Here's how the part is built. I have some questions about the finished solid (model axes, mm). Face numbers are marked on the shaded views. A direction names the side the tool comes from. Round coordinates to 2 decimals unless told otherwise and drop trailing zeros. Write each loop counter-clockwise with the first axis right and the second up, starting at its lowest first coordinate (ties: lowest second). Pieces come first, ordered by that corner, then holes. Notation, with made-up numbers: (-17, 30) - (4, 30) arc R33 ccw to (4, 62) - close; hole circle Ø6 at (38, 76). An arc over 180 degrees is marked (long way). Use one line per item in the form item = value. Start each with the question number.
1. I want a section at B-B, the plane y = -14.45. List the corners of the cut face in (x, z) for me, plus the area to 3 significant figures.
2. I want a section at D-D, the plane x = 12.5. List the corners of the cut face in (y, z) for me.
3. If I drill on line 1 along Y through (x, z) = (4, 3.05); line 2 along X through (y, z) = (-80, 105.25); line 3 along Y through (x, z) = (22, 2.75), over which ranges is the centre line in solid material (lowest first)?
4. I want a section at C-C, the plane z = 14.5. List the corners of the cut face in (x, y) for me.
5. Which directions (+Z, -Z, +X, -X, +Y, -Y) give clear straight access to the entire face, cutting with the end or side of a thin tool? Please do the marked faces 1 and 2.
6. I want a section at A-A, the plane x = 22. List the corners of the cut face in (y, z) for me, plus the area to 3 significant figures.
7. Will these pins go through, and if not, where does the flat tip stop? pin 1 (1.2 mm diameter, centred on x = 11.5, z = 3, fed in from -Y); pin 2 (2 mm diameter, centred on x = 4, y = -4.45, fed in from +Z) (3 decimals); pin 3 (10 mm diameter, centred on x = 35, z = 14.5, fed in from +Y); pin 4 (3 mm diameter, centred on x = 26.5, y = -51.5, fed in from -Z).
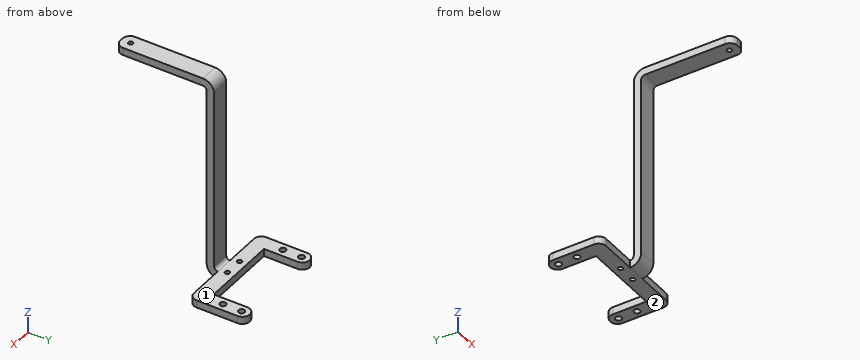
```python
from build123d import *

# Parameters (mm, degrees)
EXTRUDE_1_DEPTH                  = 3
SHEET_METAL_1_OUTLINE_W          = 8
SHEET_METAL_1_OUTLINE_H          = 1
SHEET_METAL_1_DEPTH              = 57.5
SHEET_METAL_1_2_OUTLINE_W        = 22
SHEET_METAL_1_2_OUTLINE_H        = 1
SHEET_METAL_1_2_DEPTH            = 8
SHEET_START                      = 49.5
SHEET_METAL_1_3_OUTLINE_W        = 22
SHEET_METAL_1_3_OUTLINE_H        = 1
SHEET_METAL_1_3_DEPTH            = 8
SM_EDGE_FLANGE_1_DEPTH           = 10
SM_EDGE_FLANGE_2_STRIP_W         = 20
SM_EDGE_FLANGE_2_STRIP_H         = 4
SM_EDGE_FLANGE_2_STRIP_CUT_DEPTH = 10
SM_EDGE_FLANGE_2_DEPTH           = 10
FILLET_1_R                       = 4
M4X0_7_1_D                       = 3.3
M3X0_5_1_D                       = 2.5
M3X0_5_2_D                       = 2.5


# Read off the part's stored shape, not the designer's step: 轉換-實體1
# Sheet-metal steps are written as plain solids
with BuildPart() as part:
    # Sketch 1 → 填料-伸長1 (new body)
    with BuildSketch(Plane.XY):
        Polygon((8, 0), (8, -22), (49.5, -22), (49.5, 0), (57.5, 0), (57.5, -30), (8, -30), (0, -30), (0, 0), align=None)
    extrude(amount=EXTRUDE_1_DEPTH)

    # Sheet Metal 1 outline → Sheet Metal 1 (add)
    with BuildSketch(Plane.YZ):
        with Locations((-26, 3.5)):
            Rectangle(SHEET_METAL_1_OUTLINE_W, SHEET_METAL_1_OUTLINE_H)
    extrude(amount=SHEET_METAL_1_DEPTH)

    # Sheet Metal 1 2 outline → Sheet Metal 1 2 (add)
    with BuildSketch(Plane.YZ):
        with Locations((-11, 3.5)):
            Rectangle(SHEET_METAL_1_2_OUTLINE_W, SHEET_METAL_1_2_OUTLINE_H)
    extrude(amount=SHEET_METAL_1_2_DEPTH)

    # Sheet Metal 1 3 outline → Sheet Metal 1 3 (add)
    with BuildSketch(Plane.YZ.offset(SHEET_START)):
        with Locations((-11, 3.5)):
            Rectangle(SHEET_METAL_1_3_OUTLINE_W, SHEET_METAL_1_3_OUTLINE_H)
    extrude(amount=SHEET_METAL_1_3_DEPTH)

    # 邊線-凸緣1 section (across the edge) → 邊線-凸緣1 (add)
    with BuildSketch(Plane(origin=(23.75, -32, 4), x_dir=(0, 1, 0), z_dir=(1, 0, 0))):
        with BuildLine():
            Line((-4, 2), (-4, 104.15))
            Line((-4, 104.15), (0, 104.15))
            Line((0, 104.15), (0, 2))
            ThreePointArc((0, 2), (0.585786438, 0.585786438), (2, 0))
            Line((2, 0), (2, -4))
            ThreePointArc((2, -4), (-2.242640687, -2.242640687), (-4, 2))
        make_face()
    extrude(amount=SM_EDGE_FLANGE_1_DEPTH)

    # 邊線-凸緣2 strip (across the edge) → 邊線-凸緣2 strip cut (cut)
    with BuildSketch(Plane(origin=(33.75, -36, 108.15), x_dir=(0, 0, -1), z_dir=(-1, 0, 0))):
        with Locations((-4, -2)):
            Rectangle(SM_EDGE_FLANGE_2_STRIP_W, SM_EDGE_FLANGE_2_STRIP_H)
    extrude(amount=SM_EDGE_FLANGE_2_STRIP_CUT_DEPTH, mode=Mode.SUBTRACT)

    # 邊線-凸緣2 section (across the edge) → 邊線-凸緣2 (add)
    with BuildSketch(Plane(origin=(33.75, -36, 108.15), x_dir=(0, 0, -1), z_dir=(-1, 0, 0))):
        with BuildLine():
            Line((0, 2), (0, 49))
            Line((0, 49), (4, 49))
            Line((4, 49), (4, 2))
            ThreePointArc((4, 2), (4.585786438, 0.585786438), (6, 0))
            Line((6, 0), (6, -4))
            ThreePointArc((6, -4), (1.757359313, -2.242640687), (0, 2))
        make_face()
    extrude(amount=SM_EDGE_FLANGE_2_DEPTH)

    # 圓角1
    fillet_1_edges = [part.edges().sort_by_distance(p)[0] for p in [
        (0, -30, 2),
        (57.5, -30, 2),
        (57.5, 0, 2),
        (49.5, 0, 2),
        (8, 0, 2),
        (0, 0, 2),
        (33.75, -85, 106.15),
        (23.75, -85, 106.15),
    ]]
    fillet(fillet_1_edges, radius=FILLET_1_R - 0.0001)  # a hair under: the kernel refuses the full size

    # M4x0.7 螺紋孔1 (through all)
    with Locations(Plane(origin=(53.5, -4.45, 0), x_dir=(-1, 0, 0), z_dir=(0, 0, -1))):
        with Locations((0, 0), (0, -10), (49.5, -10), (49.5, 0)):
            Hole(M4X0_7_1_D / 2)

    # M3x0.5 螺紋孔1 (through all)
    with Locations(Plane(origin=(28.75, -80, 104.15), x_dir=(-1, 0, 0), z_dir=(0, 0, -1))):
        with Locations((0, 0)):
            Hole(M3X0_5_1_D / 2)

    # M3x0.5 螺紋孔2 (through all)
    with Locations(Plane(origin=(22, -26, 0), x_dir=(-1, 0, 0), z_dir=(0, 0, -1))):
        with Locations((0, 0), (-10, 0)):
            Hole(M3X0_5_2_D / 2)


solid = part.part
```
Model answer:
q1.outline = (0, 0) - (2.35, 0) - (2.35, 4) - (0, 4) - close; (5.65, 0) - (8, 0) - (8, 4) - (5.65, 4) - close; (49.5, 0) - (51.85, 0) - (51.85, 4) - (49.5, 4) - close; (55.15, 0) - (57.5, 0) - (57.5, 4) - (55.15, 4) - close
q1.area = 37.6 mm2
q2.outline = (-30, 0) - (-22, 0) - (-22, 4) - (-30, 4) - close
q3.line_1 = -30 to -16.1, -12.8 to -6.1, -2.8 to 0
q3.line_2 = 23.75 to 27.5, 30 to 33.75
q3.line_3 = -30 to -27.25, -24.75 to -22
q4.outline = (23.75, -36) - (33.75, -36) - (33.75, -32) - (23.75, -32) - close
q5.face_1 = +Z, +X, -X, +Y
q5.face_2 = -Z, +X, -X, +Y, -Y
q6.outline = (-30, 0) - (-27.25, 0) - (-27.25, 4) - (-30, 4) - close; (-24.75, 0) - (-22, 0) - (-22, 4) - (-24.75, 4) - close
q6.area = 22.0 mm2
q7.pin_1 = -30
q7.pin_2 = through
q7.pin_3 = -32
q7.pin_4 = 104.15
